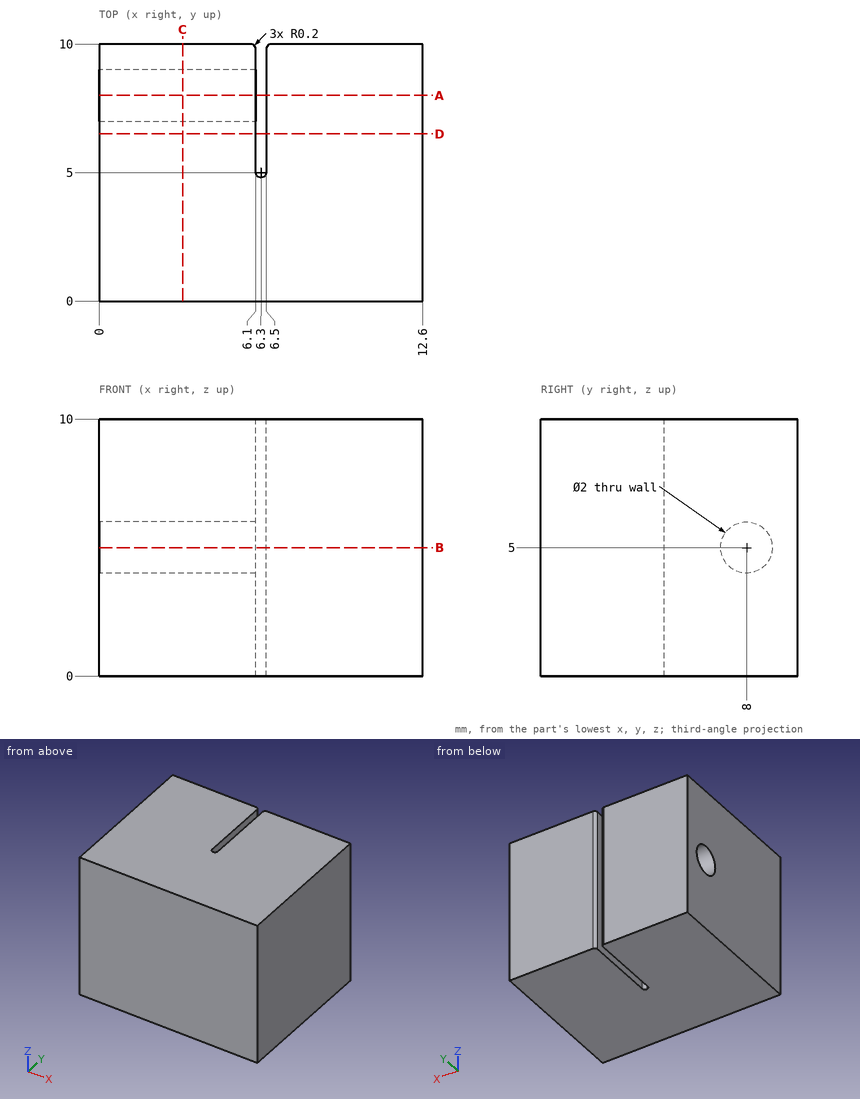
Input: dimensioned drawing with shaded views. Units: mm. Origin: part minimum x, y, z. Give positions to 0.01 mm unless a question says otherwise; leave off trailing zeros. Write each loop counter-clockwise with the first axis right and the second up, starting at its lowest first coordinate (ties: lowest second). Pieces come first, ordered by that corner, then holes. Notation, with made-up numbers: (2, 1) -> (20, 1) arc R17 ccw to (20, 25) -> close; hole circle Ø1 at (71.25, 20). An arc over 180 degrees is marked (long way). Answer as a JSON object with one key per item and string values.
1. Cut plane D-D on y = 6.5. Output: boundary loops of the cut face in (x, z).
Ans:
{"outline": "(0, 0) -> (6.1, 0) -> (6.1, 10) -> (0, 10) -> close; (6.5, 0) -> (12.6, 0) -> (12.6, 10) -> (6.5, 10) -> close"}
2. Ray query, probe 1 along Z at (x, y) = (3.25, 8); probe 2 along X at (y, z) = (5.5, 9.75). Return the intervals inside material, ascending. Write a range as from..to.
Ans:
{"probe 1": "z = 0..4, 6..10", "probe 2": "x = 0..6.1, 6.5..12.6"}
3. Cut plane A-A on y = 8. Output: boundary loops of the cut face in (x, z).
Ans:
{"outline": "(0, 0) -> (6.1, 0) -> (6.1, 4) -> (0, 4) -> close; (0, 6) -> (6.1, 6) -> (6.1, 10) -> (0, 10) -> close; (6.5, 0) -> (12.6, 0) -> (12.6, 10) -> (6.5, 10) -> close"}
4. Cut plane C-C on x = 3.25. Output: boundary loops of the cut face in (y, z).
Ans:
{"outline": "(0, 0) -> (10, 0) -> (10, 10) -> (0, 10) -> close; hole circle Ø2 at (8, 5)"}
5. Cut plane B-B on z = 5. Output: boundary loops of the cut face in (x, y).
Ans:
{"outline": "(0, 0) -> (12.6, 0) -> (12.6, 10) -> (6.7, 10) arc R0.2 ccw to (6.5, 9.8) -> (6.5, 5) arc R0.2 cw to (6.3, 4.8) arc R0.2 cw to (6.1, 5) -> (6.1, 7) -> (0, 7) -> close; (0, 9) -> (6.1, 9) -> (6.1, 9.8) arc R0.2 ccw to (5.9, 10) -> (0, 10) -> close"}
